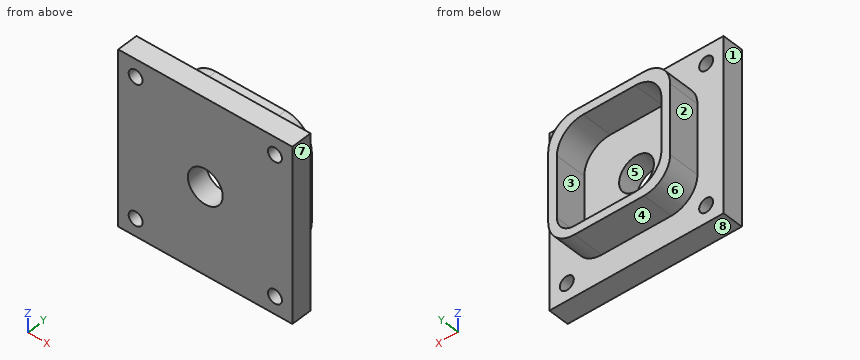
```python
from build123d import *

# Parameters (mm, degrees)
F0_W     = 100
F0_H     = 100
F1_DEPTH = 12
F2_R     = 4
F2_R_2   = 10
F3_DEPTH = 12
F5_DEPTH = 18


with BuildPart() as f1:
    # F0 (on Front) → F1 (new body)
    with BuildSketch(Plane.XZ):
        Rectangle(F0_W, F0_H)
    extrude(amount=F1_DEPTH)

    # F2 (on face) → F3 (cut)
    with BuildSketch(Plane(origin=(0, 0, 0), x_dir=(-1, 0, 0), z_dir=(0, 1, 0))):
        with Locations((-40, -40)):
            Circle(F2_R)
        with Locations((-40, 40)):
            Circle(F2_R)
        with Locations((40, -40)):
            Circle(F2_R)
        with Locations((40, 40)):
            Circle(F2_R)
        Circle(F2_R_2)
    extrude(amount=-F3_DEPTH, mode=Mode.SUBTRACT)

    # F4 (on face) → F5 (join)
    with BuildSketch(Plane(origin=(0, 0, 0), x_dir=(-1, 0, 0), z_dir=(0, 1, 0))):
        with BuildLine():
            ThreePointArc((-35, -20), (-30.606602, -30.606602), (-20, -35))
            Line((-20, -35), (20, -35))
            ThreePointArc((20, -35), (30.606602, -30.606602), (35, -20))
            Line((35, -20), (35, 20))
            ThreePointArc((35, 20), (30.606602, 30.606602), (20, 35))
            Line((20, 35), (-20, 35))
            ThreePointArc((-20, 35), (-30.606602, 30.606602), (-35, 20))
            Line((-35, 20), (-35, -20))
        make_face()
        with BuildLine():
            Line((15, -30), (-20, -30))
            ThreePointArc((-20, -30), (-27.071068, -27.071068), (-30, -20))
            Line((-30, -20), (-30, 15))
            ThreePointArc((-30, 15), (-25.606602, 25.606602), (-15, 30))
            Line((-15, 30), (15, 30))
            ThreePointArc((15, 30), (25.606602, 25.606602), (30, 15))
            Line((30, 15), (30, -15))
            ThreePointArc((30, -15), (25.606602, -25.606602), (15, -30))
        make_face(mode=Mode.SUBTRACT)
    extrude(amount=F5_DEPTH)


solid = f1.part
```
Can you work these out from the model? Positions are in its coordinate system, mm. Face numbers are marked on the shaded views. A direction names the side the tool comes from. Round coordinates to 2 decimals unless told otherwise and drop trailing zeros. Loops run counter-clockwise (first coordinate to the right, second up) from the corner with the lowest first, then second, coordinate; pieces in that order, holes last. Notation, with made-up numbers: M -39,53.25 L 13,53.25 A15 cw 13,66.25 Z; hole C -12.5,76 d2. An arc over 180 degrees is marked long. Write item = value, one per line. Start each with the question number.
(1) If we mould it in two halves opening along X, with no side actions, what happens to the marked faces 5, 6, 7 and 8? For each: released by +X, released by -X, zero draft, split by the parting line, or undercut.
(2) Suppose I cut it at A-A on z = -40. Write out the boundary of the cut face in (x, y).
(3) I need wall thicknesses on line 1 along X through (y, z) = (11.25, 14.5); line 2 along Z through (x, y) = (0, -6); line 3 along Z through (x, y) = (-40, -6.5). Which ranges of each line are inside material? Lowest first, please.
(4) Suppose I cut it at C-C on x = 0. Write out the boundary of the cut face in (y, z).
(5) Which directions (+Z, -Z, +X, -X, +Y, -Y) give clear straight access to the entire face, cutting with the end or side of a thin tool? Please do the marked faces 1, 2, 3 and 4.
(6) I'm going to push flat-ended pins straight in: P1, Ø9, axis at y = 6.5, z = 6.5, coming from the +X side; P2, Ø3, axis at x = -13, y = 13, coming from the +Z side; P3, Ø10, axis at x = 5.5, y = 12, coming from the -Z side. Where does each tip first touch, or does it pass through?
(7) Suppose I cut it at D-D on z = -4. Write out the boundary of the cut face in (x, y), plus the area to 3 significant figures.
(8) Suppose I cut it at B-B on y = 6.5. Write out the boundary of the cut face in (x, z).
Answer block:
q1.face_5 = undercut
q1.face_6 = released by -X
q1.face_7 = released by +X
q1.face_8 = zero draft
q2.outline = M -50,-12 L -44,-12 L -44,0 L -50,0 Z; M -36,-12 L 36,-12 L 36,0 L -36,0 Z; M 44,-12 L 50,-12 L 50,0 L 44,0 Z
q3.line_1 = -35 to -30, 30 to 35
q3.line_2 = -50 to -10, 10 to 50
q3.line_3 = -50 to -44, -36 to 36, 44 to 50
q4.outline = M -12,-50 L 0,-50 L 0,-35 L 18,-35 L 18,-30 L 0,-30 L 0,-10 L -12,-10 Z; M -12,10 L 0,10 L 0,30 L 18,30 L 18,35 L 0,35 L 0,50 L -12,50 Z
q5.face_1 = +Z, -Z, -X, +Y, -Y
q5.face_2 = +Z, -Z, -X, +Y
q5.face_3 = +Y
q5.face_4 = -Z, +X, -X, +Y
q6.P1 = 35
q6.P2 = 35
q6.P3 = -35
q7.outline = M -50,-12 L -9.17,-12 L -9.17,0 L -30,0 L -30,18 L -35,18 L -35,0 L -50,0 Z; M 9.17,-12 L 50,-12 L 50,0 L 35,0 L 35,18 L 30,18 L 30,0 L 9.17,0 Z
q7.area = 1,160 mm²
q8.outline = M -35,-20 A15 ccw -20,-35 L 20,-35 A15 ccw 35,-20 L 35,20 A15 ccw 20,35 L -20,35 A15 ccw -35,20 Z; hole M -30,-15 A15 ccw -15,-30 L 20,-30 A10 ccw 30,-20 L 30,15 A15 ccw 15,30 L -15,30 A15 ccw -30,15 Z
